The listing builds one solid part. Answer for the finished solid, in the listing's coordinates (mm). Face numbers are marked on the shaded views. A direction names the side the tool comes from. Coordinates: 2 decimals unless noted, no trailing zeros. Order: outer loops, then holes, each group sorted by start corner. A loop starts at its lowest first (then second) coordinate and runs counter-clockwise, first axis right, second up. Notation, with made-up numbers: (21, -5.5) -> (41, -5.5) arc R30 ccw to (41, 28.5) -> close; hole circle Ø1 at (58.5, 10). An arc over 180 degrees is marked (long way). Answer in a Markdown table with one row per item. Add a question column.
```python
from build123d import *

# Parameters (mm, degrees)
SKETCH1_W                   = 254
SKETCH1_H                   = 152.4
BOSS_EXTRUDE1_DEPTH         = 3
SKETCH2_W                   = 254
SKETCH2_H                   = 177.8
BOSS_EXTRUDE2_DEPTH         = 3
SKETCH3_W                   = 210
SKETCH3_H                   = 30
BOSS_EXTRUDE3_DEPTH         = 110
SKETCH4_W                   = 104
SKETCH4_H                   = 27
SKETCH4_W_2                 = 100
CUT_EXTRUDE1_DEPTH          = 110
F_6_CLEARANCE_HOLE1_D       = 3.7973
F_6_CLEARANCE_HOLE1_DEPTH   = 3
M3_CLEARANCE_HOLE1_D        = 3.4
M3_CLEARANCE_HOLE1_DEPTH    = 3
M3_CLEARANCE_HOLE2_D        = 3.4
M3_CLEARANCE_HOLE2_DEPTH    = 3
M3_CLEARANCE_HOLE3_D        = 3.4
M3_CLEARANCE_HOLE3_DEPTH    = 3
F_1_4_CLEARANCE_HOLE1_D     = 6.7564
F_1_4_CLEARANCE_HOLE1_DEPTH = 3
M3_CLEARANCE_HOLE4_D        = 3.4
CUT_EXTRUDE2_REACH          = 347.477
SKETCH26_W                  = 38.1
SKETCH26_H                  = 174.8


with BuildPart() as part:
    # Sketch1 → Boss-Extrude1 (new body)
    with BuildSketch(Plane(origin=(0, 0, 0), x_dir=(1, 0, 0), z_dir=(0, 1, 0))):
        with Locations((127, -76.2)):
            Rectangle(SKETCH1_W, SKETCH1_H)
    extrude(amount=BOSS_EXTRUDE1_DEPTH)

    # Sketch2 → Boss-Extrude2 (add)
    with BuildSketch(Plane(origin=(0, 0, 0), x_dir=(-1, 0, 0), z_dir=(0, 0, -1))):
        with Locations((-127, 88.9)):
            Rectangle(SKETCH2_W, SKETCH2_H)
    extrude(amount=BOSS_EXTRUDE2_DEPTH)

    # Sketch3 → Boss-Extrude3 (add)
    with BuildSketch(Plane.XY):
        with Locations((112.553077541, 94.2404)):
            Rectangle(SKETCH3_W, SKETCH3_H)
    extrude(amount=BOSS_EXTRUDE3_DEPTH)

    # Sketch4 → Cut-Extrude1 (cut)
    with BuildSketch(Plane.XY.offset(110)):
        with Locations((162.553077541, 95.7404)):
            Rectangle(SKETCH4_W, SKETCH4_H)
        with Locations((57.553077541, 95.7404)):
            Rectangle(SKETCH4_W_2, SKETCH4_H)
    extrude(amount=-CUT_EXTRUDE1_DEPTH, mode=Mode.SUBTRACT)

    # #6 Clearance Hole1
    with Locations(Plane(origin=(0, 0, 0), x_dir=(-1, 0, 0), z_dir=(0, -1, 0))):
        with Locations((-40.113, -11.985), (-40.113, -135.429), (-220.453, -11.985), (-198.863, -135.429)):
            Hole(F_6_CLEARANCE_HOLE1_D / 2, depth=F_6_CLEARANCE_HOLE1_DEPTH)

    # M3 Clearance Hole1
    with Locations(Plane(origin=(0, 79.2404, 0), x_dir=(-1, 0, 0), z_dir=(0, -1, 0))):
        with Locations((-62.053077541, -28.5), (-62.053077541, -83.5), (-169.053077541, -83.5), (-169.053077541, -28.5)):
            Hole(M3_CLEARANCE_HOLE1_D / 2, depth=M3_CLEARANCE_HOLE1_DEPTH)

    # M3 Clearance Hole2
    with Locations(Plane(origin=(110.553077541, 0, 0), x_dir=(0, 0, -1), z_dir=(1, 0, 0))):
        with Locations((-94, 97.2404), (-20.506947641, 93.829062569)):
            Hole(M3_CLEARANCE_HOLE2_D / 2, depth=M3_CLEARANCE_HOLE2_DEPTH)

    # M3 Clearance Hole3
    with Locations(Plane(origin=(217.553077541, 0, 0), x_dir=(0, 0, -1), z_dir=(1, 0, 0))):
        with Locations((-94, 97.2404), (-20, 97.2404)):
            Hole(M3_CLEARANCE_HOLE3_D / 2, depth=M3_CLEARANCE_HOLE3_DEPTH)

    # 1/4 Clearance Hole1
    with Locations(Plane(origin=(0, 3, 0), x_dir=(1, 0, 0), z_dir=(0, 1, 0))):
        with Locations((244.489784516, -272.977286046), (241.3, -139.7), (12.7, -139.7), (12.7, -12.7), (241.3, -12.7), (127, -139.7)):
            Hole(F_1_4_CLEARANCE_HOLE1_D / 2, depth=F_1_4_CLEARANCE_HOLE1_DEPTH)

    # M3 Clearance Hole4 (through all)
    with Locations(Plane.XY):
        with Locations((17.553077541, 155.5904), (17.553077541, 130.5904), (200.553077541, 155.5904), (200.553077541, 130.5904)):
            Hole(M3_CLEARANCE_HOLE4_D / 2)

    # Sketch26 → Cut-Extrude2 (cut, up to next)
    with BuildSketch(Plane.XY, mode=Mode.PRIVATE) as cut_extrude2_sk1:
        with Locations((234.95, 90.4)):
            Rectangle(SKETCH26_W, SKETCH26_H)
    cut_extrude2_tool1 = extrude(cut_extrude2_sk1.sketch, amount=-CUT_EXTRUDE2_REACH, mode=Mode.PRIVATE) & part.part
    add(cut_extrude2_tool1.solids().sort_by_distance((234.95, 90.4, 0))[0], mode=Mode.SUBTRACT)


solid = part.part
```
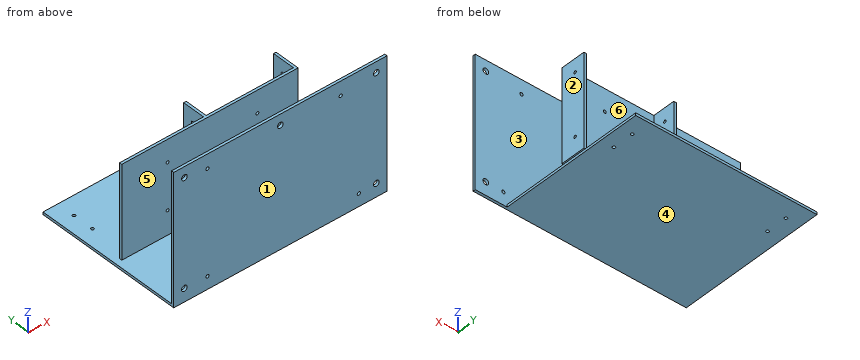
Q1. Straight lines are drawn through the part: line 1 (Y direction, x = 127, z = 13); line 2 (X direction, y = 80, z = 83); line 3 (X direction, y = 95, z = 107.5). For each, find the intervals that lie inside material, in ascending order.
Q2. A cutting plane is placed at A-A (z = 67). Determine the outline of the cut face in (x, y), then the cut area to 3 significant figures.
Q3. For the marked faces 1 and 2, determine the directions among +Z, -Z, +X, -X, +Y, -Y from which every point of the face is accessible in a straight line to the end or side of a thin tool.
Q4. Determine the mould class of the marked faces 3, 4, 5 and 6 for opening direction Y: +Y half, -Y half, draft (parallel to the pull), parting line (faces both ways), or undercut.
Q5. Given pin 1 (2.5 mm diameter, centred on y = 77, z = -2, fed in from +X); pin 2 (5 mm diameter, centred on y = 85, z = 22, fed in from -X); pin 3 (10 mm diameter, centred on x = 118.5, y = 157.5, fed in from +Z); pin 4 (4 mm diameter, centred on x = 241.3, z = 12.7, fed in from -Y), each flat-ended and moving along its own axis, determine where each tip first touches the part or whether it passes through.
Q6. A cutting plane is placed at D-D (y = 75.5). Determine the outline of the cut face in (x, z).
Q7. A cutting plane is placed at B-B (x = 12.7). Determine the outline of the cut face in (y, z), then the cut area to 3 significant figures.
Q8. A cutting plane is placed at C-C (x = 241.3). Determine the outline of the cut face in (y, z), then the cut area to 3 significant figures.
Returned:
| question | item | result |
|---|---|---|
| 1 | line 1 | y = 0 to 3, 79.24 to 82.24 |
| 1 | line 2 | x = 7.55 to 60.43, 63.68 to 167.43, 170.68 to 217.55 |
| 1 | line 3 | x = 107.55 to 110.55, 214.55 to 217.55 |
| 2 | outline | (0, 0) -> (254, 0) -> (254, 3) -> (0, 3) -> close; (7.55, 79.24) -> (217.55, 79.24) -> (217.55, 109.24) -> (214.55, 109.24) -> (214.55, 82.24) -> (110.55, 82.24) -> (110.55, 109.24) -> (107.55, 109.24) -> (107.55, 82.24) -> (7.55, 82.24) -> close |
| 2 | area | 1,550 mm² |
| 3 | face 1 | +Z, -Z, +X, -X, -Y |
| 3 | face 2 | +Z, -Z, +X, +Y |
| 4 | face 3 | undercut |
| 4 | face 4 | draft |
| 4 | face 5 | undercut |
| 4 | face 6 | +Y half |
| 5 | pin 1 | stops at x = 215.9 |
| 5 | pin 2 | stops at x = 107.55 |
| 5 | pin 3 | stops at z = 0 |
| 5 | pin 4 | passes through |
| 6 | outline | (0, -3) -> (215.9, -3) -> (215.9, 0) -> (0, 0) -> close |
| 7 | outline | (0, -3) -> (177.8, -3) -> (177.8, 0) -> (82.24, 0) -> (82.24, 110) -> (79.24, 110) -> (79.24, 0) -> (3, 0) -> (3, 9.32) -> (0, 9.32) -> close; (0, 16.08) -> (3, 16.08) -> (3, 136.32) -> (0, 136.32) -> close; (0, 143.08) -> (3, 143.08) -> (3, 152.4) -> (0, 152.4) -> close |
| 7 | area | 1,280 mm² |
| 8 | outline | (0, -3) -> (3, -3) -> (3, 9.32) -> (0, 9.32) -> close; (0, 16.08) -> (3, 16.08) -> (3, 136.32) -> (0, 136.32) -> close; (0, 143.08) -> (3, 143.08) -> (3, 152.4) -> (0, 152.4) -> close |
| 8 | area | 426 mm² |
